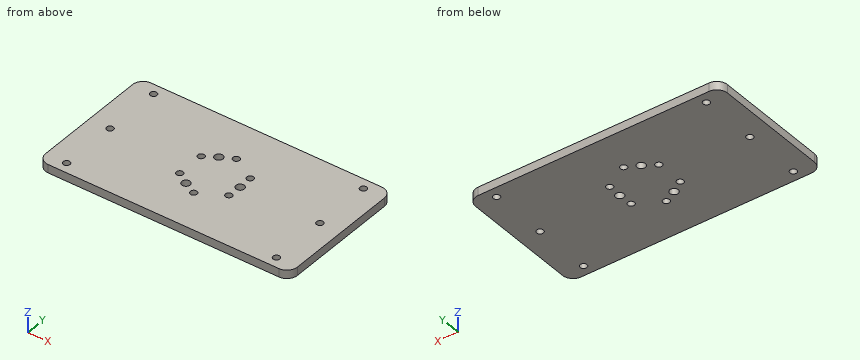
```python
from build123d import *

# Parameters (mm, degrees)
SKETCH_1_W          = 120
SKETCH_1_H          = 65
EXTRUDE_1_DEPTH     = 4
SKETCH_2_R          = 1.6
CUT_EXTRUDE_1_DEPTH = 137.53204752
FILLET_1_R          = 5
SKETCH_4_R          = 2
SKETCH_4_R_2        = 1.6
CUT_EXTRUDE_3_DEPTH = 12.5


with BuildPart() as part:
    # 草图1 → 凸台-拉伸1 (new body)
    with BuildSketch(Plane.XY):
        with Locations((60, -32.5)):
            Rectangle(SKETCH_1_W, SKETCH_1_H)
    extrude(amount=EXTRUDE_1_DEPTH)

    # 草图2 → 切除-拉伸1 (cut, through all)
    with BuildSketch(Plane.XY.offset(4)):
        with Locations((10, -5)):
            Circle(SKETCH_2_R)
        with Locations((10, -32.5)):
            Circle(SKETCH_2_R)
        with Locations((10, -60)):
            Circle(SKETCH_2_R)
        with Locations(Location((110, -60, 0), (0, 0, 180))):
            Circle(SKETCH_2_R)
        with Locations(Location((110, -32.5, 0), (0, 0, 180))):
            Circle(SKETCH_2_R)
        with Locations(Location((110, -5, 0), (0, 0, 180))):
            Circle(SKETCH_2_R)
    extrude(amount=-CUT_EXTRUDE_1_DEPTH, mode=Mode.SUBTRACT)

    # 圆角1
    fillet_1_edges = [part.edges().sort_by_distance(p)[0] for p in [
        (0, 0, 2),
        (120, 0, 2),
        (120, -65, 2),
        (0, -65, 2),
    ]]
    fillet(fillet_1_edges, radius=FILLET_1_R)

    # 草图4 → 切除-拉伸3 (cut)
    with BuildSketch(Plane.XY.offset(4)):
        with Locations((72, -32.5)):
            Circle(SKETCH_4_R)
        with Locations((60, -19)):
            Circle(SKETCH_4_R_2)
        with Locations((71.691342951, -25.75)):
            Circle(SKETCH_4_R_2)
        with Locations((71.691342951, -39.25)):
            Circle(SKETCH_4_R_2)
        with Locations((60, -46)):
            Circle(SKETCH_4_R_2)
        with Locations((48.308657049, -39.25)):
            Circle(SKETCH_4_R_2)
        with Locations((48.308657049, -25.75)):
            Circle(SKETCH_4_R_2)
        with Locations((54, -42.892304845)):
            Circle(SKETCH_4_R)
        with Locations((54, -22.107695155)):
            Circle(SKETCH_4_R)
    extrude(amount=-CUT_EXTRUDE_3_DEPTH, mode=Mode.SUBTRACT)


solid = part.part
```
Input: part model. Units: mm. Frame: model coordinates. Round coordinates to 2 decimals unless told otherwise and drop trailing zeros. Order: outer loops, then holes, each group sorted by start corner. A loop starts at its lowest first (then second) coordinate and runs counter-clockwise, first axis right, second up. Notation, with made-up numbers: (6.25, 77.25) - (38.25, 77.25) arc R17 ccw to (38.25, 105.25) - close; hole circle Ø6 at (71, 13.25). An arc over 180 degrees is marked (long way). One line per question, with ' | ' between items. Start each with the question number.
1) Cut plane C-C, the plane x = 110. Return the cut outline in (y, z), then the cut area to 3 significant figures.
2) Cut plane B-B, the plane y = -46. Return the cut outline in (x, z), then the cut area to 3 significant figures.
3) Cut plane D-D, the plane y = -39.25. Return the cut outline in (x, z), then the cut area to 3 significant figures.
4) Ray query, probe 1 along Y at (x, z) = (54, 1.2); probe 2 along Y at (x, z) = (60, 2); probe 3 along Y at (x, z) = (110, 2.45). Return the intervals inside material, ascending.
5) Contact query for a flat-ended pin moving along its axis: P1, Ø4, axis at x = 71.69, y = -25.75, coming from the +Z side. Output: stop coordinate, or through.
6) Cut plane A-A, the plane x = 54. Return the cut outline in (y, z).
Worked out:
1) outline: (-65, 0) - (-61.6, 0) - (-61.6, 4) - (-65, 4) - close; (-58.4, 0) - (-34.1, 0) - (-34.1, 4) - (-58.4, 4) - close; (-30.9, 0) - (-6.6, 0) - (-6.6, 4) - (-30.9, 4) - close; (-3.4, 0) - (0, 0) - (0, 4) - (-3.4, 4) - close | area: 222 mm^2
2) outline: (0, 0) - (58.4, 0) - (58.4, 4) - (0, 4) - close; (61.6, 0) - (120, 0) - (120, 4) - (61.6, 4) - close | area: 467 mm^2
3) outline: (0, 0) - (46.71, 0) - (46.71, 4) - (0, 4) - close; (49.91, 0) - (70.09, 0) - (70.09, 4) - (49.91, 4) - close; (73.29, 0) - (120, 0) - (120, 4) - (73.29, 4) - close | area: 454 mm^2
4) probe 1: y = -65 to -44.89, -40.89 to -24.11, -20.11 to 0 | probe 2: y = -65 to -47.6, -44.4 to -20.6, -17.4 to 0 | probe 3: y = -65 to -61.6, -58.4 to -34.1, -30.9 to -6.6, -3.4 to 0
5) P1: stops at z = 4
6) outline: (-65, 0) - (-44.89, 0) - (-44.89, 4) - (-65, 4) - close; (-40.89, 0) - (-24.11, 0) - (-24.11, 4) - (-40.89, 4) - close; (-20.11, 0) - (0, 0) - (0, 4) - (-20.11, 4) - close
